```python
from build123d import *

# Parameters (mm, degrees)
ESTRUSIONE_ESTRUSIONE1_DEPTH = 80
FORO_6_5_6_5_1_D             = 6.5
FORO_6_5_6_5_2_D             = 6.5
FORO_6_5_6_5_2_DEPTH         = 5
FORO_6_5_6_5_2_TIP           = 1.952797012
TAGLIO_ESTRUSIONE1_REACH     = 108.771
SCHIZZO8_R                   = 1.75
TAGLIO_ESTRUSIONE2_REACH     = 108.771
SCHIZZO9_R                   = 1.75
SMUSSO1_SIZE                 = 3


with BuildPart() as part:
    # Schizzo1 → Estrusione-Estrusione1 (new body)
    with BuildSketch(Plane.XY):
        Polygon((0, 0), (0, 50), (5, 50), (5, 5), (50, 5), (50, 0), align=None)
    extrude(amount=ESTRUSIONE_ESTRUSIONE1_DEPTH)

    # Foro Ø6.5 (6.5)-1 (through all)
    with Locations(Plane(origin=(0, 0, 0), x_dir=(-1, 0, 0), z_dir=(0, -1, 0))):
        with Locations((-17, -72), (-42, -72)):
            Hole(FORO_6_5_6_5_1_D / 2)

    # Foro Ø6.5 (6.5)-2
    with Locations(Plane.ZY):
        with Locations((72, 42), (72, 17)):
            Hole(FORO_6_5_6_5_2_D / 2, depth=FORO_6_5_6_5_2_DEPTH)
            with Locations((0, 0, -(FORO_6_5_6_5_2_DEPTH + FORO_6_5_6_5_2_TIP / 2))):  # 118° drill point
                Cone(0, FORO_6_5_6_5_2_D / 2, FORO_6_5_6_5_2_TIP, mode=Mode.SUBTRACT)

    # Schizzo8 → Taglio-Estrusione1 (cut, up to next)
    with BuildSketch(Plane.XZ, mode=Mode.PRIVATE) as taglio_estrusione1_sk1:
        with Locations((20, 10)):
            Circle(SCHIZZO8_R)
    taglio_estrusione1_tool1 = extrude(taglio_estrusione1_sk1.sketch, amount=-TAGLIO_ESTRUSIONE1_REACH, mode=Mode.PRIVATE) & part.part
    # Schizzo8 → Taglio-Estrusione1 (cut, up to next)
    with BuildSketch(Plane.XZ, mode=Mode.PRIVATE) as taglio_estrusione1_sk2:
        with Locations((20, 30)):
            Circle(SCHIZZO8_R)
    taglio_estrusione1_tool2 = extrude(taglio_estrusione1_sk2.sketch, amount=-TAGLIO_ESTRUSIONE1_REACH, mode=Mode.PRIVATE) & part.part
    # Schizzo8 → Taglio-Estrusione1 (cut, up to next)
    with BuildSketch(Plane.XZ, mode=Mode.PRIVATE) as taglio_estrusione1_sk3:
        with Locations((40, 30)):
            Circle(SCHIZZO8_R)
    taglio_estrusione1_tool3 = extrude(taglio_estrusione1_sk3.sketch, amount=-TAGLIO_ESTRUSIONE1_REACH, mode=Mode.PRIVATE) & part.part
    # Schizzo8 → Taglio-Estrusione1 (cut, up to next)
    with BuildSketch(Plane.XZ, mode=Mode.PRIVATE) as taglio_estrusione1_sk4:
        with Locations((40, 10)):
            Circle(SCHIZZO8_R)
    taglio_estrusione1_tool4 = extrude(taglio_estrusione1_sk4.sketch, amount=-TAGLIO_ESTRUSIONE1_REACH, mode=Mode.PRIVATE) & part.part
    add(taglio_estrusione1_tool1.solids().sort_by_distance((20, 0, 10))[0], mode=Mode.SUBTRACT)
    add(taglio_estrusione1_tool2.solids().sort_by_distance((20, 0, 30))[0], mode=Mode.SUBTRACT)
    add(taglio_estrusione1_tool3.solids().sort_by_distance((40, 0, 30))[0], mode=Mode.SUBTRACT)
    add(taglio_estrusione1_tool4.solids().sort_by_distance((40, 0, 10))[0], mode=Mode.SUBTRACT)

    # Schizzo9 → Taglio-Estrusione2 (cut, up to next)
    with BuildSketch(Plane.ZY, mode=Mode.PRIVATE) as taglio_estrusione2_sk1:
        with Locations((30, 40)):
            Circle(SCHIZZO9_R)
    taglio_estrusione2_tool1 = extrude(taglio_estrusione2_sk1.sketch, amount=-TAGLIO_ESTRUSIONE2_REACH, mode=Mode.PRIVATE) & part.part
    # Schizzo9 → Taglio-Estrusione2 (cut, up to next)
    with BuildSketch(Plane.ZY, mode=Mode.PRIVATE) as taglio_estrusione2_sk2:
        with Locations((50, 40)):
            Circle(SCHIZZO9_R)
    taglio_estrusione2_tool2 = extrude(taglio_estrusione2_sk2.sketch, amount=-TAGLIO_ESTRUSIONE2_REACH, mode=Mode.PRIVATE) & part.part
    # Schizzo9 → Taglio-Estrusione2 (cut, up to next)
    with BuildSketch(Plane.ZY, mode=Mode.PRIVATE) as taglio_estrusione2_sk3:
        with Locations((50, 20)):
            Circle(SCHIZZO9_R)
    taglio_estrusione2_tool3 = extrude(taglio_estrusione2_sk3.sketch, amount=-TAGLIO_ESTRUSIONE2_REACH, mode=Mode.PRIVATE) & part.part
    # Schizzo9 → Taglio-Estrusione2 (cut, up to next)
    with BuildSketch(Plane.ZY, mode=Mode.PRIVATE) as taglio_estrusione2_sk4:
        with Locations((30, 20)):
            Circle(SCHIZZO9_R)
    taglio_estrusione2_tool4 = extrude(taglio_estrusione2_sk4.sketch, amount=-TAGLIO_ESTRUSIONE2_REACH, mode=Mode.PRIVATE) & part.part
    add(taglio_estrusione2_tool1.solids().sort_by_distance((0, 40, 30))[0], mode=Mode.SUBTRACT)
    add(taglio_estrusione2_tool2.solids().sort_by_distance((0, 40, 50))[0], mode=Mode.SUBTRACT)
    add(taglio_estrusione2_tool3.solids().sort_by_distance((0, 20, 50))[0], mode=Mode.SUBTRACT)
    add(taglio_estrusione2_tool4.solids().sort_by_distance((0, 20, 30))[0], mode=Mode.SUBTRACT)

    # Smusso1
    smusso1_edges = [part.edges().sort_by_distance(p)[0] for p in [
        (2.5, 50, 80),
        (2.5, 50, 0),
        (50, 2.5, 80),
        (50, 2.5, 0),
    ]]
    chamfer(smusso1_edges, length=SMUSSO1_SIZE)


solid = part.part
```
The listing builds one solid part. Answer for the finished solid, in the listing's coordinates (mm). A direction names the side the tool comes from. Give positions to 0.01 mm unless a question says otherwise; leave off trailing zeros. Order: outer loops, then holes, each group sorted by start corner. A loop starts at its lowest first (then second) coordinate and runs counter-clockwise, first axis right, second up. Notation, with made-up numbers: (69.5, 41) -> (119.5, 41) arc R31 cw to (119.5, 73) -> close; hole circle Ø4 at (6, 74). An arc over 180 degrees is marked (long way). One line per item, written item: value.
1) Find section A-A, the plane z = 50. Determine the outline of the cut face in (x, y).
Reported:
outline: (0, 0) -> (50, 0) -> (50, 5) -> (5, 5) -> (5, 18.25) -> (0, 18.25) -> close; (0, 21.75) -> (5, 21.75) -> (5, 38.25) -> (0, 38.25) -> close; (0, 41.75) -> (5, 41.75) -> (5, 50) -> (0, 50) -> close
2) Find section C-C, the plane y = 17. Determine the outline of the cut face in (x, z).
Reported:
outline: (0, 0) -> (5, 0) -> (5, 68.75) -> (0, 68.75) -> close; (0, 75.25) -> (5, 75.25) -> (5, 80) -> (0, 80) -> close
3) Find section B-B, the plane z = 72. Determine the outline of the cut face in (x, y).
Reported:
outline: (0, 0) -> (13.75, 0) -> (13.75, 5) -> (5, 5) -> (5, 13.75) -> (0, 13.75) -> close; (0, 20.25) -> (5, 20.25) -> (5, 38.75) -> (0, 38.75) -> close; (0, 45.25) -> (5, 45.25) -> (5, 50) -> (0, 50) -> close; (20.25, 0) -> (38.75, 0) -> (38.75, 5) -> (20.25, 5) -> close; (45.25, 0) -> (50, 0) -> (50, 5) -> (45.25, 5) -> close
4) A tool of negligible diameter and unlimited length cuts with its end or side. For faces 1 (the cylindrical face through (41.669, 2.465, 10.526)), 2 (the flat face through (5, 28, 39)), from which of +Z, -Z, +X, -X, +Y, -Y can it reach the whole face along a straight path? Write none if from no direction.
Reported:
face 1: +Y, -Y
face 2: +Z, -Z, +X, +Y
5) Determine the mould class of faces 3 (the cylindrical face through (18.71, 2.46, 11.18)), 4 (the flat face through (49, 3, 2)), 5 (the flat face through (49, 3, 78)), 6 (the flat face through (25, 0, 39)) for opening direction Z: pulls with the +Z half, pulls with the -Z half, needs draft (parallel to the pull), parting line crosses it, or undercut.
Reported:
face 3: undercut
face 4: pulls with the -Z half
face 5: pulls with the +Z half
face 6: needs draft
6) Find the intervals of material crossed by line 1 (Y direction, x = 1, z = 50); line 2 (Z direction, x = 40, y = 2); line 3 (Z direction, x = 17, y = 3), in increasing order.
Reported:
line 1: y = 0 to 18.25, 21.75 to 38.25, 41.75 to 50
line 2: z = 0 to 8.25, 11.75 to 28.25, 31.75 to 69.44, 74.56 to 80
line 3: z = 0 to 68.75, 75.25 to 80
7) Flat-ended cylindrical pins translate along their axes: P1, Ø5.5, axis at y = 20, z = 30, coming from the +X side; P2, Ø7.5, axis at x = 17, z = 72, coming from the +Y side. Find the tip coordinate at first contact, or state that the pin passes through.
Reported:
P1: stops at x = 5
P2: stops at y = 5
